Build history of the part. All positions in model axes, mm. A direction names the side the tool comes from. Round coordinates to 2 decimals unless told otherwise and drop trailing zeros. Write each loop counter-clockwise with the first axis right and the second up, starting at its lowest first coordinate (ties: lowest second). Pieces come first, ordered by that corner, then holes.
Item 1: 3-axis set-ups, long thin cutter, end or side, ignore diameter. For faces 1 (the flat face through (-41, 5, 19)), 2 (the flat face through (49, 45.56, -7)), 3 (the cylindrical face through (-43.5, 19.9, 39)): which of +Z, -Z, +X, -X, +Y, -Y reach the whole face in a straight line?
Item 2: Wall check: probe 1 along Z at (x, y) = (22.5, 38); probe 2 along X at (y, z) = (30, 6); probe 3 along Y at (x, z) = (28, -39). Give the ranges that are in metal, low to high.
Item 3: Band-saw the part on A-A, the plane x = 28. Write the cut outline in (y, z).
Item 4: Drop flat-ended pins along their axis: pin 1 Ø2 at (x, z) = (48.5, -5.5) entering from +Y; pin 2 Ø1.5 at (x, z) = (-41, 18.5) entering from +Y; pin 3 Ø4.5 at (x, y) = (49.5, 53) entering from -Z. Give the stop position or say it passes through.
Item 5: Band-saw the part on C-C, the plane y = 67.5. Write the cut outline in (x, z), then the cut area to 3 significant figures.
Item 6: Mould opens along X. For faces 4 (the flat face through (49, 32.5, -5)), 5 (the cylindrical face through (-43.5, 9.93, -30.07)), 6 (the flat face through (-33, 85, -39)) say: +X half, -X half, draft (parallel to the pull), parting line (faces both ways), or undercut.
Item 7: Band-saw the part on B-B, the plane y = 77.5. Write the cut outline in (x, z).
Item 8: Band-saw the part on D-D, the plane z = 34. Write the cut outline in (x, y), then the cut area to 3 significant figures.
```python
from build123d import *

# Parameters (mm, degrees)
SKETCH1_W           = 102
SKETCH1_H           = 82
BOSS_EXTRUDE1_DEPTH = 5
SKETCH2_W           = 102
SKETCH2_H           = 82
SKETCH2_W_2         = 94
SKETCH2_H_2         = 74
BOSS_EXTRUDE2_DEPTH = 70
CUT_EXTRUDE1_REACH  = 84
SKETCH9_W           = 20
SKETCH9_H           = 15
SKETCH9_W_2         = 10
SKETCH9_H_2         = 13
CUT_EXTRUDE7_DEPTH  = 10
SKETCH10_R          = 5
SKETCH10_R_2        = 4.5
BOSS_EXTRUDE5_DEPTH = 10
SKETCH11_R          = 1.5
CUT_EXTRUDE8_DEPTH  = 10
SKETCH13_W          = 10
SKETCH13_H          = 5
BOSS_EXTRUDE6_DEPTH = 20
SKETCH14_R          = 2.5
CUT_EXTRUDE9_DEPTH  = 10


with BuildPart() as part:
    # Sketch1 → Boss-Extrude1 (new body)
    with BuildSketch(Plane(origin=(0, 0, 0), x_dir=(1, 0, 0), z_dir=(0, 1, 0))):
        Rectangle(SKETCH1_W, SKETCH1_H)
    extrude(amount=BOSS_EXTRUDE1_DEPTH)

    # Sketch2 → Boss-Extrude2 (add)
    with BuildSketch(Plane(origin=(0, 5, 0), x_dir=(1, 0, 0), z_dir=(0, 1, 0))):
        Rectangle(SKETCH2_W, SKETCH2_H)
        Rectangle(SKETCH2_W_2, SKETCH2_H_2, mode=Mode.SUBTRACT)
    extrude(amount=BOSS_EXTRUDE2_DEPTH)

    # Sketch4 → Cut-Extrude1 (cut, up to next)
    with BuildSketch(Plane.XY.offset(41), mode=Mode.PRIVATE) as cut_extrude1_sk1:
        with BuildLine():
            Line((-38.5, 25), (-28.5, 25))
            ThreePointArc((-28.5, 25), (-23.5, 20), (-28.5, 15))
            Line((-28.5, 15), (-38.5, 15))
            ThreePointArc((-38.5, 15), (-43.5, 20), (-38.5, 25))
        make_face()
    cut_extrude1_tool1 = extrude(cut_extrude1_sk1.sketch, amount=-CUT_EXTRUDE1_REACH, mode=Mode.PRIVATE) & part.part
    add(cut_extrude1_tool1.solids().sort_by_distance((-33.5, 20, 41))[0], mode=Mode.SUBTRACT)

    # Sketch9 → Cut-Extrude7 (cut)
    with BuildSketch(Plane(origin=(51, 0, 0), x_dir=(0, 0, -1), z_dir=(1, 0, 0))):
        with Locations((5.5, 25)):
            Rectangle(SKETCH9_W, SKETCH9_H)
        with Locations((7.375245753, 52.06044871)):
            Rectangle(SKETCH9_W_2, SKETCH9_H_2)
    extrude(amount=-CUT_EXTRUDE7_DEPTH, mode=Mode.SUBTRACT)

    # Sketch10 → Boss-Extrude5 (add)
    with BuildSketch(Plane(origin=(0, 5, 0), x_dir=(1, 0, 0), z_dir=(0, 1, 0))):
        with Locations((17, -20)):
            Circle(SKETCH10_R)
        with Locations((-40.991198651, -18.989614408)):
            Circle(SKETCH10_R)
        with Locations((15.99137867, 29)):
            Circle(SKETCH10_R)
        with Locations((-42, 30)):
            Circle(SKETCH10_R_2)
    extrude(amount=BOSS_EXTRUDE5_DEPTH)

    # Sketch11 → Cut-Extrude8 (cut)
    with BuildSketch(Plane(origin=(0, 5, 0), x_dir=(1, 0, 0), z_dir=(0, 1, 0))):
        with Locations((-42, 30)):
            Circle(SKETCH11_R)
        with Locations((15.99137867, 29)):
            Circle(SKETCH11_R)
        with Locations((-40.991198651, -18.989614408)):
            Circle(SKETCH11_R)
        with Locations((17, -20)):
            Circle(SKETCH11_R)
    extrude(amount=CUT_EXTRUDE8_DEPTH, mode=Mode.SUBTRACT)

    # Sketch13 → Boss-Extrude6 (add)
    with BuildSketch(Plane(origin=(0, 75, 0), x_dir=(1, 0, 0), z_dir=(0, 1, 0))):
        with Locations((-28, 39.5)):
            Rectangle(SKETCH13_W, SKETCH13_H)
        with Locations((28, 39.5)):
            Rectangle(SKETCH13_W, SKETCH13_H)
    extrude(amount=BOSS_EXTRUDE6_DEPTH)

    # Sketch14 → Cut-Extrude9 (cut)
    with BuildSketch(Plane.XY.offset(-37)):
        with Locations((-28, 90)):
            Circle(SKETCH14_R)
        with Locations((28, 90)):
            Circle(SKETCH14_R)
    extrude(amount=-CUT_EXTRUDE9_DEPTH, mode=Mode.SUBTRACT)


solid = part.part
```
Results:
1. face 1: +Y
1. face 2: +X
1. face 3: +Z
2. probe 1: z = -41 to -37, 37 to 41
2. probe 2: x = -51 to -47, 47 to 51
2. probe 3: y = 0 to 87.5, 92.5 to 95
3. outline: (0, -41) - (75, -41) - (75, -42) - (87.5, -42) - (87.5, -37) - (5, -37) - (5, 37) - (75, 37) - (75, 41) - (0, 41) - close; (92.5, -42) - (95, -42) - (95, -37) - (92.5, -37) - close
4. pin 1: stops at y = 75
4. pin 2: stops at y = 5
4. pin 3: stops at z = -41
5. outline: (-51, -41) - (51, -41) - (51, 41) - (-51, 41) - close; hole (-47, -37) - (47, -37) - (47, 37) - (-47, 37) - close
5. area: 1,410 mm2
6. face 4: draft
6. face 5: undercut
6. face 6: -X half
7. outline: (-33, -42) - (-23, -42) - (-23, -37) - (-33, -37) - close; (23, -42) - (33, -42) - (33, -37) - (23, -37) - close
8. outline: (-51, 0) - (51, 0) - (51, 75) - (47, 75) - (47, 5) - (-47, 5) - (-47, 75) - (-51, 75) - close
8. area: 1,070 mm2
